For this review, take the finished solid that the model builds, in its own axes (mm). A direction names the side the tool comes from. Give positions to 0.01 mm unless a question says otherwise; leave off trailing zeros. Order: outer loops, then holes, each group sorted by start corner. A loop starts at its lowest first (then second) coordinate and runs counter-clockwise, first axis right, second up.
from build123d import *

# Parameters (mm, degrees)
SKETCH1_R           = 1.5875
BOSS_EXTRUDE1_DEPTH = 6.35


with BuildPart() as part:
    # Sketch1 → Boss-Extrude1 (new, symmetric)
    with BuildSketch(Plane.XY):
        with BuildLine():
            Line((-6.857967121, 4.433224129), (-53.175519737, 12.600258336))
            ThreePointArc((-53.175519737, 12.600258336), (-54.999856137, 11.322844236), (-56.277270236, 13.147180636))
            Line((-56.277270236, 13.147180636), (-58.257319182, 13.496316688))
            Line((-58.257319182, 13.496316688), (-59.35998511, 7.242787457))
            Line((-59.35998511, 7.242787457), (-7.960633049, -1.820305103))
            ThreePointArc((-7.960633049, -1.820305103), (-4.365043482, -6.901563925), (1.766856325, -7.9726663))
            Line((1.766856325, -7.9726663), (36.881050722, -0.047144418))
            Line((36.881050722, -0.047144418), (34.635185978, 2.889025961))
            ThreePointArc((34.635185978, 2.889025961), (44.961162175, 6.595254431), (55.860821822, 5.346521684))
            ThreePointArc((55.860821822, 5.346521684), (48.726273767, 11.088641723), (39.595789676, 11.801367988))
            Line((39.595789676, 11.801367988), (6.869791404, 4.414878852))
            ThreePointArc((6.869791404, 4.414878852), (0.010912869, 8.166092708), (-6.857967121, 4.433224129))
        make_face()
        Circle(SKETCH1_R, mode=Mode.SUBTRACT)
    extrude(amount=BOSS_EXTRUDE1_DEPTH, both=True)


solid = part.part
1) We need section D-D on x = -50.5. Give the boundary of the cut face in (y, z), then the cut area to 3 significant figures.
Answer sheet:
outline: (5.68, -6.35) - (12.13, -6.35) - (12.13, 6.35) - (5.68, 6.35) - close
area: 81.9 mm2
2) Clearance check with flat-ended pins moving along their axes: pin 1 (1.5 mm diameter, centred on y = 10.5, z = 4, fed in from -X); pin 2 (2 mm diameter, centred on y = 0, z = -4.5, fed in from +X); pin 3 (2 mm diameter, centred on x = -8, z = 0.5, fed in from +Y). State where each tip first meets the part, or that it passes through.
Answer sheet:
pin 1: stops at x = -58.92
pin 2: stops at x = 36.88
pin 3: stops at y = 4.81
3) To check wall thickness, follow line 1 (Y direction, x = 0, z = -1.25); line 2 (Y direction, x = 23.5, z = -3); line 3 (Y direction, x = 16, z = -3.75). State the ranges of each line that lie inside material, in increasing order.
Answer sheet:
line 1: y = -8.17 to -1.59, 1.59 to 8.17
line 2: y = -3.07 to 8.17
line 3: y = -4.76 to 6.48
4) Tool access review of faces 1 (the face through (-29.69, 8.46, 0.09)), 2 (the face through (-58.8, 10.41, 0.09)), 3 (the face through (35.774, 1.4, 0.089)): name each direction out of +Z, -Z, +X, -X, +Y, -Y from which nothing blocks a thin tool from reaching the whole face with its end or side.
Answer sheet:
face 1: +Z, -Z, +Y
face 2: +Z, -Z, -X, +Y
face 3: +Z, -Z, +X
5) Draft analysis for pull direction X (two halves, no side actions). For faces 4 (the face through (-57.25, 13.32, 0.09)), 5 (the face through (-54.966, 11.317, 0.089)), 6 (the face through (-3, 3, -6.35)), state which applies: +X half, -X half, draft (parallel to the pull), parting line (faces both ways), or undercut.
Answer sheet:
face 4: +X half
face 5: undercut
face 6: draft
6) We need section C-C on y = -3.5. Give the boundary of the cut face in (x, z), then the cut area to 3 significant figures.
Answer sheet:
outline: (-7.38, -6.35) - (21.58, -6.35) - (21.58, 6.35) - (-7.38, 6.35) - close
area: 368 mm2
7) We need section B-B on x = 0. Give the boundary of the cut face in (y, z), then the cut area to 3 significant figures.
Answer sheet:
outline: (-8.17, -6.35) - (-1.59, -6.35) - (-1.59, 6.35) - (-8.17, 6.35) - close; (1.59, -6.35) - (8.17, -6.35) - (8.17, 6.35) - (1.59, 6.35) - close
area: 167 mm2
8) We need section A-A on z = -4.5. Give the boundary of the cut face in (x, y) (1 decimal).
Answer sheet:
outline: (-59.4, 7.2) - (-8, -1.8) arc R8.2 ccw to (1.8, -8) - (36.9, 0) - (34.6, 2.9) arc R24.1 cw to (55.9, 5.3) arc R15.5 ccw to (39.6, 11.8) - (6.9, 4.4) arc R8.2 ccw to (-6.9, 4.4) - (-53.2, 12.6) arc R1.6 cw to (-56.3, 13.1) - (-58.3, 13.5) - close; hole circle Ø3.2 at (0, 0)
